from build123d import *

# Parameters (mm, degrees)
SKETCH_1_R               = 10.5
EXTRUDE_1_DEPTH          = 28
SKETCH_2_R               = 12.5
EXTRUDE_2_DEPTH          = 2
FILLET_1_R               = 1
CHAMFER_1_SIZE           = 1
CUT_EXTRUDE_1_DEPTH      = 35.820970729
CUT_EXTRUDE_1_DEPTH_BACK = 35.820970729
SKETCH_3_R               = 4


with BuildPart() as part:
    # Эскиз1 → Бобышка-Вытянуть1 (new body)
    with BuildSketch(Plane(origin=(0, 0, 0), x_dir=(1, 0, 0), z_dir=(0, 1, 0))):
        with Locations(Location((0, 0, 0), (0, 0, 270))):
            Circle(SKETCH_1_R)
    extrude(amount=EXTRUDE_1_DEPTH)

    # Эскиз2 → Бобышка-Вытянуть2 (add)
    with BuildSketch(Plane(origin=(0, 28, 0), x_dir=(1, 0, 0), z_dir=(0, 1, 0))):
        with Locations(Location((0, 0, 0), (0, 0, 270))):
            Circle(SKETCH_2_R)
    extrude(amount=EXTRUDE_2_DEPTH)

    # Скругление1
    fillet_1_edges = [part.edges().sort_by_distance(p)[0] for p in [
        (0, 30, -12.5),
    ]]
    fillet(fillet_1_edges, radius=FILLET_1_R)

    # Фаска1
    chamfer_1_edges = [part.edges().sort_by_distance(p)[0] for p in [
        (0, 0, -10.5),
    ]]
    chamfer(chamfer_1_edges, length=CHAMFER_1_SIZE)

    # Эскиз3 → Вырез-Вытянуть1 (cut, two sides: drawn at the far end of the back side and taken through both)
    with BuildSketch(Plane.XY.offset(-CUT_EXTRUDE_1_DEPTH_BACK)):
        with Locations(Location((0, 13, 0), (0, 0, 89.999999999))):
            Circle(SKETCH_3_R)
    extrude(amount=CUT_EXTRUDE_1_DEPTH + CUT_EXTRUDE_1_DEPTH_BACK, mode=Mode.SUBTRACT)


solid = part.part
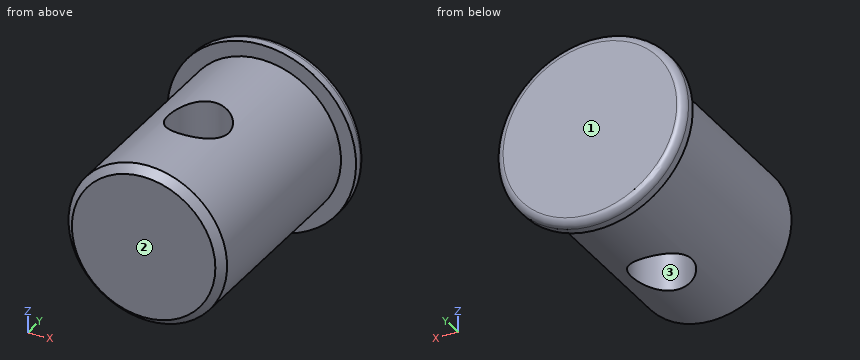
Geometry: final body of the model. Coordinates: model frame, mm. Face numbers are marked on the shaded views. Coordinates: 2 decimals unless noted, no trailing zeros. Loops run counter-clockwise (first coordinate to the right, second up) from the corner with the lowest first, then second, coordinate; pieces in that order, holes last. Notation, with made-up numbers: M 25.25,43 L 70.25,43 A8 cw 70.25,58 Z; hole C 67,25.5 d11. An arc over 180 degrees is marked long. One line per item, written item: value. Start each with the question number.
1) Material intervals for L1, parallel to X at y = 13, z = 5; L2, parallel to X at y = 26.25, z = 0.25; L3, parallel to X at y = 13, z = -4.5, sorted ascending. Write a range as from..to.
2) Cut plane D-D (y = 13). Return loops of the section in (x, z).
3) Draft query along Y for the marked faces 1, 2 and 3. Return one class per face: released by +Y, released by -Y, zero draft, split by the parting line, or undercut.
4) Cut plane B-B (z = 0). Return loops of the section in (x, y), then the cut area to 3 significant figures.
5) Pin query (flat end, axial travel): P1, Ø4, axis at x = -4.5, y = 13.5, coming from the +Z side; P2, Ø1.5, axis at x = 1.5, y = 20.5, coming from the +Z side; P3, Ø2, axis at x = -6.5, y = 14.5, coming from the -Z side. Return the tip coordinate at first contact, or that it passes through.
6) Cut plane C-C (y = 16.5). Return loops of the section in (x, z).
7) Cut plane A-A (x = 0). Return loops of the section in (y, z).
Evaluation:
1. L1: -9.23..-4, 4..9.23
1. L2: -10.5..10.5
1. L3: -9.49..-4, 4..9.49
2. outline: M -4,-9.71 L -4,9.71 A10.5 ccw Z; M 4,-9.71 A10.5 ccw 4,9.71 Z
3. face 1: released by +Y
3. face 2: released by -Y
3. face 3: undercut
4. outline: M -12.5,28 L -10.5,28 L -10.5,1 L -9.5,0 L 9.5,0 L 10.5,1 L 10.5,28 L 12.5,28 L 12.5,29 A1 ccw 11.5,30 L -11.5,30 A1 ccw -12.5,29 Z; hole C 0,13 d8
4. area: 586 mm^2
5. P1: z = 9.94
5. P2: z = 10.47
5. P3: z = -8.94
6. outline: M -1.94,-10.32 L -1.94,10.32 A10.5 ccw Z; M 1.94,-10.32 A10.5 ccw 1.94,10.32 Z
7. outline: M 0,-9.5 L 1,-10.5 L 9,-10.5 L 9,10.5 L 1,10.5 L 0,9.5 Z; M 17,-10.5 L 28,-10.5 L 28,-12.5 L 29,-12.5 A1 ccw 30,-11.5 L 30,11.5 A1 ccw 29,12.5 L 28,12.5 L 28,10.5 L 17,10.5 Z
